from build123d import *

# Parameters (mm, degrees)
ESTRUSIONE_ESTRUSIONE2_DEPTH = 6
SCHIZZO2_W                   = 25
SCHIZZO2_H                   = 36
ESTRUSIONE_ESTRUSIONE3_DEPTH = 8
TAGLIO_ESTRUSIONE1_DEPTH     = 15
TAGLIO_ESTRUSIONE2_DEPTH     = 10.5
ESTRUSIONE_ESTRUSIONE5_DEPTH = 10
ESTRUSIONE_ESTRUSIONE6_DEPTH = 5
SCHIZZO8_R                   = 1.75
TAGLIO_ESTRUSIONE3_DEPTH     = 17
SCHIZZO9_R                   = 5
SCHIZZO9_R_2                 = 3
ESTRUSIONE_ESTRUSIONE7_DEPTH = 10
RACCORDO1_R                  = 3
SMUSSO1_SIZE                 = 0.5
SMUSSO2_SIZE                 = 1.86


with BuildPart() as part:
    # Schizzo1 → Estrusione-Estrusione2 (new body)
    with BuildSketch(Plane.XY):
        Polygon((-8, -60), (-8, 60), (52, 105), (97, 105), (137, 50), (137, -50), (97, -105), (52, -105), align=None)
    extrude(amount=ESTRUSIONE_ESTRUSIONE2_DEPTH)

    # Schizzo2 → Estrusione-Estrusione3 (add)
    with BuildSketch(Plane(origin=(0, 0, 0), x_dir=(-1, 0, 0), z_dir=(0, 0, -1))):
        with Locations((-4.5, -42)):
            Rectangle(SCHIZZO2_W, SCHIZZO2_H)
        with Locations((-4.5, 42)):
            Rectangle(SCHIZZO2_W, SCHIZZO2_H)
    extrude(amount=ESTRUSIONE_ESTRUSIONE3_DEPTH)

    # Schizzo3 → Taglio-Estrusione1 (cut, through all)
    with BuildSketch(Plane(origin=(0, 0, 6), x_dir=(-1, 0, 0), z_dir=(0, 0, -1))):
        Polygon((-52, 105), (-44, 99), (-52, 99), align=None)
        Polygon((-52, -105), (-44, -99), (-52, -99), align=None)
    extrude(amount=TAGLIO_ESTRUSIONE1_DEPTH, mode=Mode.SUBTRACT)

    # Schizzo4 → Taglio-Estrusione2 (cut)
    with BuildSketch(Plane(origin=(0, 0, -8), x_dir=(-1, 0, 0), z_dir=(0, 0, -1))):
        with BuildLine():
            Line((2.85, 30.0132503), (2.85, 31.8867497))
            ThreePointArc((2.85, 31.8867497), (-3, 30.95), (2.85, 30.0132503))
        make_face()
        with BuildLine():
            Line((2.85, -30.0132503), (2.85, -31.8867497))
            ThreePointArc((2.85, -31.8867497), (-3, -30.95), (2.85, -30.0132503))
        make_face()
    extrude(amount=-TAGLIO_ESTRUSIONE2_DEPTH, mode=Mode.SUBTRACT)

    # Schizzo6 → Estrusione-Estrusione5 (add)
    with BuildSketch(Plane(origin=(0, 0, 0), x_dir=(-1, 0, 0), z_dir=(0, 0, -1))):
        with BuildLine():
            Line((-65, -5.25), (-75, -5.25))
            ThreePointArc((-75, -5.25), (-80.25, 0), (-75, 5.25))
            Line((-75, 5.25), (-65, 5.25))
            ThreePointArc((-65, 5.25), (-59.75, 0), (-65, -5.25))
        make_face()
        with BuildLine():
            Line((-65, -3.25), (-75, -3.25))
            ThreePointArc((-75, -3.25), (-78.25, 0), (-75, 3.25))
            Line((-75, 3.25), (-65, 3.25))
            ThreePointArc((-65, 3.25), (-61.75, 0), (-65, -3.25))
        make_face(mode=Mode.SUBTRACT)
        with BuildLine():
            Line((-97.192473147, 53.28), (-99.588351187, 53.28))
            ThreePointArc((-99.588351187, 53.28), (-101.00256475, 52.694213562), (-101.588351187, 51.28))
            Line((-101.588351187, 51.28), (-101.588351187, 45.28))
            ThreePointArc((-101.588351187, 45.28), (-101.00256475, 43.865786438), (-99.588351187, 43.28))
            Line((-99.588351187, 43.28), (-88.338351187, 43.28))
            ThreePointArc((-88.338351187, 43.28), (-86.924137625, 43.865786438), (-86.338351187, 45.28))
            Line((-86.338351187, 45.28), (-86.338351187, 46.58848156))
            ThreePointArc((-86.338351187, 46.58848156), (-86.715866817, 47.757902129), (-87.705895655, 48.485848156))
            Line((-87.705895655, 48.485848156), (-92.067947473, 49.939865428))
            ThreePointArc((-92.067947473, 49.939865428), (-92.312116926, 50.004445295), (-92.562478503, 50.037737372))
            ThreePointArc((-92.562478503, 50.037737372), (-94.238582432, 50.643407271), (-95.343283829, 52.041904762))
            ThreePointArc((-95.343283829, 52.041904762), (-96.079775867, 52.94189794), (-97.192473147, 53.28))
        make_face()
        with BuildLine():
            Line((-97.192473147, -53.28), (-99.588351187, -53.28))
            ThreePointArc((-99.588351187, -53.28), (-101.00256475, -52.694213562), (-101.588351187, -51.28))
            Line((-101.588351187, -51.28), (-101.588351187, -45.28))
            ThreePointArc((-101.588351187, -45.28), (-101.00256475, -43.865786438), (-99.588351187, -43.28))
            Line((-99.588351187, -43.28), (-88.338351187, -43.28))
            ThreePointArc((-88.338351187, -43.28), (-86.924137625, -43.865786438), (-86.338351187, -45.28))
            Line((-86.338351187, -45.28), (-86.338351187, -46.58848156))
            ThreePointArc((-86.338351187, -46.58848156), (-86.715866817, -47.757902129), (-87.705895655, -48.485848156))
            Line((-87.705895655, -48.485848156), (-92.067947473, -49.939865428))
            ThreePointArc((-92.067947473, -49.939865428), (-92.312116926, -50.004445295), (-92.562478503, -50.037737372))
            ThreePointArc((-92.562478503, -50.037737372), (-94.238582432, -50.643407271), (-95.343283829, -52.041904762))
            ThreePointArc((-95.343283829, -52.041904762), (-96.079775867, -52.94189794), (-97.192473147, -53.28))
        make_face()
        with BuildLine():
            Line((-75.270403715, -92.59965352), (-79.632455532, -94.053670792))
            ThreePointArc((-79.632455532, -94.053670792), (-80.62248437, -94.781616819), (-81, -95.951037389))
            Line((-81, -95.951037389), (-81, -96.959518948))
            ThreePointArc((-81, -96.959518948), (-80.414213562, -98.373732511), (-79, -98.959518948))
            Line((-79, -98.959518948), (-71, -98.959518948))
            ThreePointArc((-71, -98.959518948), (-68.171572875, -97.787946073), (-67, -94.959518948))
            Line((-67, -94.959518948), (-67, -91.259518948))
            ThreePointArc((-67, -91.259518948), (-67.585786438, -89.845305386), (-69, -89.259518948))
            Line((-69, -89.259518948), (-70.14587804, -89.259518948))
            ThreePointArc((-70.14587804, -89.259518948), (-71.258575321, -89.597621009), (-71.995067358, -90.497614187))
            ThreePointArc((-71.995067358, -90.497614187), (-73.099768755, -91.896111677), (-74.775872685, -92.501781576))
            ThreePointArc((-74.775872685, -92.501781576), (-75.026234261, -92.535073654), (-75.270403715, -92.59965352))
        make_face()
        with BuildLine():
            Line((-70.14587804, 89.259518948), (-69, 89.259518948))
            ThreePointArc((-69, 89.259518948), (-67.585786438, 89.845305386), (-67, 91.259518948))
            Line((-67, 91.259518948), (-67, 94.959518948))
            ThreePointArc((-67, 94.959518948), (-68.171572875, 97.787946073), (-71, 98.959518948))
            Line((-71, 98.959518948), (-79, 98.959518948))
            ThreePointArc((-79, 98.959518948), (-80.414213562, 98.373732511), (-81, 96.959518948))
            Line((-81, 96.959518948), (-81, 95.951037389))
            ThreePointArc((-81, 95.951037389), (-80.62248437, 94.781616819), (-79.632455532, 94.053670792))
            Line((-79.632455532, 94.053670792), (-75.270403715, 92.59965352))
            ThreePointArc((-75.270403715, 92.59965352), (-75.026234261, 92.535073654), (-74.775872685, 92.501781576))
            ThreePointArc((-74.775872685, 92.501781576), (-73.099768755, 91.896111677), (-71.995067358, 90.497614187))
            ThreePointArc((-71.995067358, 90.497614187), (-71.258575321, 89.597621009), (-70.14587804, 89.259518948))
        make_face()
    extrude(amount=ESTRUSIONE_ESTRUSIONE5_DEPTH)

    # Schizzo7 → Estrusione-Estrusione6 (add)
    with BuildSketch(Plane(origin=(0, 0, 0), x_dir=(-1, 0, 0), z_dir=(0, 0, -1))):
        Polygon((-52, -105), (-97, -105), (-137, -50), (-137, 50), (-97, 105), (-52, 105), (-52, 102), (-95.472326225, 102), (-134, 49.024448559), (-134, -49.024448559), (-95.472326225, -102), (-52, -102), align=None)
    extrude(amount=ESTRUSIONE_ESTRUSIONE6_DEPTH)

    # Schizzo8 → Taglio-Estrusione3 (cut, through all)
    with BuildSketch(Plane.XY.offset(6)):
        with Locations((62, 96)):
            Circle(SCHIZZO8_R)
        with Locations((109.263051754, 71.136465702)):
            Circle(SCHIZZO8_R)
        with Locations((127, 35)):
            Circle(SCHIZZO8_R)
        with Locations((127, -35)):
            Circle(SCHIZZO8_R)
        with Locations((109.263051754, -71.136465702)):
            Circle(SCHIZZO8_R)
        with Locations((62, -96)):
            Circle(SCHIZZO8_R)
        with Locations((6, -8)):
            Circle(SCHIZZO8_R)
        with Locations((6, 8)):
            Circle(SCHIZZO8_R)
        with BuildLine():
            Line((137, 20), (97, 20))
            ThreePointArc((97, 20), (89.928932188, 17.071067812), (87, 10))
            Line((87, 10), (87, -10))
            ThreePointArc((87, -10), (89.928932188, -17.071067812), (97, -20))
            Line((97, -20), (137, -20))
            Line((137, -20), (137, 20))
        make_face()
    extrude(amount=-TAGLIO_ESTRUSIONE3_DEPTH, mode=Mode.SUBTRACT)

    # Schizzo9 → Estrusione-Estrusione7 (add)
    with BuildSketch(Plane(origin=(0, 0, 0), x_dir=(-1, 0, 0), z_dir=(0, 0, -1))):
        with Locations((-60, 15.95)):
            Circle(SCHIZZO9_R)
        with Locations((-60, 15.95)):
            Circle(SCHIZZO9_R_2, mode=Mode.SUBTRACT)
        with Locations((-60, -15.95)):
            Circle(SCHIZZO9_R)
        with Locations((-60, -15.95)):
            Circle(SCHIZZO9_R_2, mode=Mode.SUBTRACT)
    extrude(amount=ESTRUSIONE_ESTRUSIONE7_DEPTH)

    # Raccordo1
    raccordo1_edges = [part.edges().sort_by_distance(p)[0] for p in [
        (70, 5.25, 0),
        (80.25, 0, 0),
        (70, -5.25, 0),
        (65, 15.95, 0),
        (65, -15.95, 0),
        (59.75, 0, 0),
    ]]
    fillet(raccordo1_edges, radius=RACCORDO1_R)

    # Smusso1
    smusso1_edges = [part.edges().sort_by_distance(p)[0] for p in [
        (61.75, 0, -10),
        (70, 3.25, -10),
        (78.25, 0, -10),
        (70, -3.25, -10),
        (63, 15.95, -10),
        (63, -15.95, -10),
        (3, -30.95, -8),
        (3, 30.95, -8),
    ]]
    chamfer(smusso1_edges, length=SMUSSO1_SIZE)

    # Smusso2
    smusso2_edges = [part.edges().sort_by_distance(p)[0] for p in [
        (60.25, 96, 6),
        (107.513051754, 71.136465702, 6),
        (125.25, 35, 6),
        (125.25, -35, 6),
        (107.513051754, -71.136465702, 6),
        (60.25, -96, 6),
        (4.25, 8, 6),
        (4.25, -8, 6),
    ]]
    chamfer(smusso2_edges, length=SMUSSO2_SIZE)


solid = part.part
The listing builds one solid part. Answer for the finished solid, in the listing's coordinates (mm). A direction names the side the tool comes from. Give positions to 0.01 mm unless a question says otherwise; leave off trailing zeros. Order: outer loops, then holes, each group sorted by start corner. A loop starts at its lowest first (then second) coordinate and runs counter-clockwise, first axis right, second up. Notation, with made-up numbers: (10.25, -23) - (63.25, -23) arc R16 ccw to (63.25, 3) - close; hole circle Ø5 at (-13.5, 70.5). An arc over 180 degrees is marked (long way). One line per item, written item: value. Start each with the question number.
1) A cutting plane is placed at B-B on y = 0. Give the vertices of the cut face in (x, z), then the cut area to 3 significant figures.
2) Find the intervals of material crossed by L1, parallel to Y at x = 62, z = 1.1; L2, parallel to Y at x = 8, z = -6.25; L3, parallel to Y at x = 6, z = 2.5, in increasing order.
3) The mould has two halves that part along Y. Classify faces 1 (the face through (137, 35, 1)), 2 (the face through (5, -60, -4)), 3 (the face through (3.133, 31.074, -7.635)): released by +Y, released by -Y, zero draft, split by the parting line, or undercut.
4) A cutting plane is placed at C-C on y = 64. Give the vertices of the cut face in (x, z), then the cut area to 3 significant figures.
5) Given pin 1 Ø8 at (y, z) = (81, 0) entering from -X; pin 2 Ø6.5 at (x, z) = (5, -4.5) entering from +Y; pin 3 Ø5 at (y, z) = (0, -6) entering from -X, each flat-ended and moving along its own axis, determine where each tip first touches the part or whether it passes through.
6) A cutting plane is placed at A-A on x = 0. Give the vertices of the cut face in (y, z), then the cut area to 3 significant figures.
7) A tool of negligible diameter and unlimited length cuts with its end or side. For faces 4 (the face through (17, 42, -4)), 5 (the face through (80.25, -0.12, -6.45)), 6 (the face through (73, 102, -2)), 7 (the face through (70, -3.25, -5)), from which of +Z, -Z, +X, -X, +Y, -Y can it reach the whole face along a straight path? Write none if from no direction.
Answer sheet:
1. outline: (-8, 0) - (56.75, 0) arc R3 cw to (59.75, -3) - (59.75, -10) - (61.25, -10) - (61.75, -9.5) - (61.75, 0) - (78.25, 0) - (78.25, -9.5) - (78.75, -10) - (80.25, -10) - (80.25, -3) arc R3 cw to (83.25, 0) - (87, 0) - (87, 6) - (-8, 6) - close
1. area: 614 mm2
2. L1: y = -105 to -97.75, -94.25 to 94.25, 97.75 to 105
2. L2: y = -60 to -24, 24 to 60
2. L3: y = -70.5 to -9.75, -6.25 to 6.25, 9.75 to 70.5
3. face 1: zero draft
3. face 2: released by -Y
3. face 3: undercut
4. outline: (-2.67, 0) - (123.11, 0) - (123.11, -5) - (126.82, -5) - (126.82, 6) - (-2.67, 6) - close
4. area: 795 mm2
5. pin 1: stops at x = 14.67
5. pin 2: stops at y = 60
5. pin 3: stops at x = 59.75
6. outline: (-66, 0) - (-60, 0) - (-60, -8) - (-34.45, -8) - (-33.95, -7.5) - (-33.95, 2.5) - (-27.95, 2.5) - (-27.95, -7.5) - (-27.45, -8) - (-24, -8) - (-24, 0) - (24, 0) - (24, -8) - (27.45, -8) - (27.95, -7.5) - (27.95, 2.5) - (33.95, 2.5) - (33.95, -7.5) - (34.45, -8) - (60, -8) - (60, 0) - (66, 0) - (66, 6) - (-66, 6) - close
6. area: 1,240 mm2
7. face 4: -Z, +Y, -Y
7. face 5: -Z, +X
7. face 6: -Z, -X
7. face 7: -Z
